Model file for the job. Use its own axes, mm. A direction names the side the tool comes from. Coordinates: 2 decimals unless noted, no trailing zeros.
Autodesk Inventor part; units mm, degrees
ref_plane "YZ Plane" through (0, 0, 0) normal (1, 0, 0) x (0, 1, 0)
ref_plane "XZ Plane" through (0, 0, 0) normal (0, 1, 0) x (-1, 0, 0)
ref_plane "XY Plane" through (0, 0, 0) normal (0, 0, 1) x (1, 0, 0)
sketch "Sketch1" plane through (0, 0, 0) normal (0, 1, 0) x (-1, 0, 0)
  line L0 (0, 0) -> (162, 0)
  line L1 (162, 0) -> (162, 120)
  line L2 (162, 120) -> (0, 120)
  line L3 (0, 120) -> (0, 0)
  line L4 (157, 120) -> (5, 120)
  line L5 (5, 120) -> (5, 130)
  line L6 (5, 130) -> (157, 130)
  line L7 (157, 130) -> (157, 120)
  line L8 (156, 0) -> (6, 0)
  line L9 (6, 0) -> (6, -10)
  line L10 (6, -10) -> (156, -10)
  line L11 (156, -10) -> (156, 0)
  dimension "d0" = 120
  dimension "d1" = 162
  dimension "d2" = 5
  dimension "d3" = 5
  dimension "d4" = 10
  dimension "d5" = 10
  dimension "d6" = 150
extrude "Extrusion1" add sketch "Sketch1" along normal blind 5
sketch "Sketch2" plane through (0, 5, 0) normal (0, 1, 0) x (1, 0, 0)
  circle A0 centre (-147, -37) radius 1.5444
  circle A1 centre (-98, -37) radius 1.5
  circle A2 centre (-98, -95) radius 1.5
  circle A3 centre (-147, -95) radius 1.5
  circle A4 centre (-28.0426, -24.3) radius 1.5
  circle A5 centre (-146.3426, -24.3) radius 1.5
  circle A6 centre (-28.7, -95) radius 1.5
  line L0 (-75, -105.8843) -> (-67, -105.8843)
  line L1 (-67, -105.8843) -> (-67, -110.8843)
  line L2 (-67, -110.8843) -> (-75, -110.8843)
  line L3 (-75, -110.8843) -> (-75, -105.8843)
  line L4 (-75, -10.8843) -> (-67, -10.8843)
  line L5 (-67, -10.8843) -> (-67, -15.8843)
  line L6 (-67, -15.8843) -> (-75, -15.8843)
  line L7 (-75, -15.8843) -> (-75, -10.8843)
  line L8 (-25, -10.8843) -> (-33, -10.8843)
  line L9 (-33, -10.8843) -> (-33, -15.8843)
  line L10 (-33, -15.8843) -> (-25, -15.8843)
  line L11 (-25, -15.8843) -> (-25, -10.8843)
  line L12 (-25, -105.8843) -> (-33, -105.8843)
  line L13 (-33, -105.8843) -> (-33, -110.8843)
  line L14 (-33, -110.8843) -> (-25, -110.8843)
  line L15 (-25, -110.8843) -> (-25, -105.8843)
  line L16 (-15, -45) -> (-10, -45)
  line L17 (-10, -45) -> (-10, -53)
  line L18 (-10, -53) -> (-15, -53)
  line L19 (-15, -53) -> (-15, -45)
  line L20 (-65, -45) -> (-60, -45)
  line L21 (-60, -45) -> (-60, -53)
  line L22 (-60, -53) -> (-65, -53)
  line L23 (-65, -53) -> (-65, -45)
  line L24 (-60, -107) -> (-65, -107)
  line L25 (-65, -107) -> (-65, -115)
  line L26 (-65, -115) -> (-60, -115)
  line L27 (-60, -115) -> (-60, -107)
  line L28 (-10, -107) -> (-15, -107)
  line L29 (-15, -107) -> (-15, -115)
  line L30 (-15, -115) -> (-10, -115)
  line L31 (-10, -115) -> (-10, -107)
  line L32 (-162, 0) -> (-162, -120)
  line L33 (-157, -130) -> (-5, -130)
  line L34 (0, -120) -> (0, 0)
  line L35 (-152, -107) -> (-147, -107)
  line L36 (-147, -107) -> (-147, -115)
  line L37 (-147, -115) -> (-152, -115)
  line L38 (-152, -115) -> (-152, -107)
  line L39 (-147, -45) -> (-152, -45)
  line L40 (-152, -45) -> (-152, -53)
  line L41 (-152, -53) -> (-147, -53)
  line L42 (-147, -53) -> (-147, -45)
  line L43 (-90.0773, -45) -> (-85.0773, -45)
  line L44 (-85.0773, -45) -> (-85.0773, -53)
  line L45 (-85.0773, -53) -> (-90.0773, -53)
  line L46 (-90.0773, -53) -> (-90.0773, -45)
  line L47 (-85, -107) -> (-90, -107)
  line L48 (-90, -107) -> (-90, -115)
  line L49 (-90, -115) -> (-85, -115)
  line L50 (-85, -115) -> (-85, -107)
  dimension "d9" = 3
  dimension "d10" = 15
  dimension "d11" = 58
  dimension "d12" = 49
  dimension "d13" = 49
  dimension "d14" = 58
  dimension "d15" = 3
  dimension "d16" = 3
  dimension "d17" = 3.0888
  dimension "d18" = 35
  dimension "d19" = 70.7
  dimension "d20" = 118.3
  dimension "d21" = 70.7
  dimension "d22" = 118.3
  dimension "d23" = 3
  dimension "d24" = 3
  dimension "d25" = 3
  dimension "d26" = 5
  dimension "d27" = 8
  dimension "d28" = 8
  dimension "d29" = 5
  dimension "d30" = 8
  dimension "d31" = 5
  dimension "d32" = 5
  dimension "d33" = 8
  dimension "d34" = 8
  dimension "d35" = 5
  dimension "d36" = 5
  dimension "d37" = 8
  dimension "d38" = 8
  dimension "d39" = 5
  dimension "d40" = 5
  dimension "d41" = 8
  dimension "d42" = 50
  dimension "d43" = 25
  dimension "d44" = 50
  dimension "d45" = 25
  dimension "d46" = 90
  dimension "d47" = 90
  dimension "d48" = 55
  dimension "d49" = 55
  dimension "d50" = 70
  dimension "d51" = 70
  dimension "d52" = 10
  dimension "d55" = 35
  dimension "d56" = 15
  dimension "d57" = 15
  dimension "d58" = 8
  dimension "d59" = 10
  dimension "d60" = 5
  dimension "d61" = 5
  dimension "d62" = 8
  dimension "d63" = 10
  dimension "d64" = 70
  dimension "d65" = 5
  dimension "d66" = 5
  dimension "d67" = 8
  dimension "d68" = 8
  dimension "d69" = 70
  dimension "d70" = 0
  dimension "d71" = 0
extrude "Extrusion2" cut sketch "Sketch2" against normal mid plane 40
sketch "Sketch4" plane through (0, 5, 0) normal (0, 1, 0) x (1, 0, 0)
  circle A0 centre (-48.4143, -2) radius 1.5
  circle A1 centre (-119.1143, -2) radius 1.5
  circle A2 centre (-119.1143, -120.3) radius 1.5
  circle A3 centre (-48.4143, -120.3) radius 1.5
  circle A4 centre (-146.3426, -24.3) radius 1.5
  circle A5 centre (-28.0426, -24.3) radius 1.5
  circle A6 centre (-28.7, -95) radius 1.5
  line L0 (-6, 10) -> (-156, 10)
  point P0 (0, 0)
  dimension "d72" = 118.3
  dimension "d73" = 70.7
  dimension "d74" = 118.3
  dimension "d75" = 70.7
  dimension "d76" = 70.7
  dimension "d77" = 118.3
  dimension "d78" = 3
  dimension "d79" = 3
  dimension "d80" = 3
  dimension "d81" = 3
  dimension "d82" = 3
  dimension "d83" = 12
  dimension "d84" = 12
extrude "Extrusion3" cut sketch "Sketch4" against normal mid plane 30 contours A0 | A1 | A2 | A3
equation "\"d2\" = d3"
equation "\"d3\" = WoodWidth"
equation "\"d7\" = WoodWidth"
equation "\"d14\" = d11"
equation "\"d16\" = d15"
equation "\"d21\" = d19"
equation "\"d22\" = d20"
equation "\"d23\" = d9"
equation "\"d24\" = d9"
equation "\"d25\" = d9"
equation "\"d45\" = d43"
equation "\"d55\" = d18"
equation "\"d57\" = d56"
equation "\"d74\" = d72"
equation "\"d75\" = d73"
equation "\"d76\" = d75"
equation "\"d77\" = d74"
equation "\"d78\" = d79"
equation "\"d80\" = d78"
equation "\"d81\" = d78"
equation "\"d82\" = d78"
equation "\"d84\" = d83"
equation "\"WoodWidth\" = 5"
equation "\"LaserWith\" = 0.3"
properties part number "BoardCarrier"
Q1. Mould opens along Z. For faces 4 (the flat face through (-80, 2, 130)), 5 (the flat face through (-3, 2, 0)), 6 (the flat face through (-156, 2, -5)), 7 (the flat face through (-71, 3, 15.884)) say: +Z half, -Z half, draft (parallel to the pull), parting line (faces both ways), or undercut.
Answers:
face 4: +Z half
face 5: -Z half
face 6: draft
face 7: undercut
Q2. Slice it at A-A (y = 2.45). Count the separate pieces of the cut face and the enclosed holes in it, and give its area (3 significant figures).
Answers:
separate pieces: 1
enclosed holes: 23
area: 21,900 mm2
Q3. Which spindle directions (+Z, -Z, +X, -X, +Y, -Y) get a long thin tool onto all of the face, cutting with end or side? Do faces 1 (the flat face through (-159, 2, 0)), 2 (the flat face through (-29, 3, 110.884)), 3 (the flat face through (-160, 2, 120)). Say none if no direction does.
Answers:
face 1: -Z, -X, +Y, -Y
face 2: +Y, -Y
face 3: +Z, -X, +Y, -Y
Q4. Drill centre lines: line 1 (X direction, y = 2.8, z = 24.3); line 2 (X direction, y = 2.95, z = 2); line 3 (Z direction, x = -150, y = 1.4). Where is each one in solid material? Low to high.
Answers:
line 1: x = -162 to -147.84, -144.84 to -29.54, -26.54 to 0
line 2: x = -162 to -120.61, -117.61 to -49.91, -46.91 to 0
line 3: z = -10 to 45, 53 to 107, 115 to 130
